from build123d import *

# Parameters (mm, degrees)
BOSS_EXTRUDE1_DEPTH = 12.7
SKETCH3_W           = 2.54
SKETCH3_H           = 5.08
CUT_EXTRUDE1_DEPTH  = 47.550334048
SKETCH4_W           = 55.88
SKETCH4_H           = 6.35
BOSS_EXTRUDE2_DEPTH = 26.67
SKETCH5_R           = 1.6
SKETCH5_W           = 31.75
SKETCH5_H           = 12.699510518
CUT_EXTRUDE3_DEPTH  = 89.325838235
CUT_EXTRUDE4_REACH  = 92.585
FILLET1_R           = 1.27
FILLET2_R           = 2.54


with BuildPart() as part:
    # Sketch2 → Boss-Extrude1 (new body)
    with BuildSketch(Plane.XY):
        with BuildLine():
            Line((-27.94, 0), (-10.7315, 0))
            ThreePointArc((-10.7315, 0), (0, -10.7315), (10.7315, 0))
            Line((10.7315, 0), (27.94, 0))
            Line((27.94, 0), (27.94, -35))
            Line((27.94, -35), (-27.94, -35))
            Line((-27.94, -35), (-27.94, 0))
        make_face()
    extrude(amount=BOSS_EXTRUDE1_DEPTH)

    # Sketch3 → Cut-Extrude1 (cut, through all)
    with BuildSketch(Plane(origin=(0, 0, 0), x_dir=(1, 0, 0), z_dir=(0, 1, 0))):
        with Locations((-21.423122, -6.35)):
            Rectangle(SKETCH3_W, SKETCH3_H)
        with Locations((21.423122, -6.35)):
            Rectangle(SKETCH3_W, SKETCH3_H)
    extrude(amount=-CUT_EXTRUDE1_DEPTH, mode=Mode.SUBTRACT)

    # Sketch4 → Boss-Extrude2 (add)
    with BuildSketch(Plane.XY.offset(12.7)):
        with Locations((0, -31.825)):
            Rectangle(SKETCH4_W, SKETCH4_H)
    extrude(amount=BOSS_EXTRUDE2_DEPTH)

    # Mirror1: part across plane


with BuildPart() as part_1:
    add(part.part)
    add(part.part.mirror(Plane(origin=(0, 0, 39.37), x_dir=(1, 0, 0), z_dir=(0, 0, -1))))

    # Sketch5 → Cut-Extrude3 (cut, through all)
    with BuildSketch(Plane(origin=(0, -28.65, 0), x_dir=(1, 0, 0), z_dir=(0, 1, 0))):
        with Locations(Location((-16.002, -28.87, 0), (0, 0, 270))):
            Circle(SKETCH5_R)
        with Locations(Location((-16.002, -49.87, 0), (0, 0, 270))):
            Circle(SKETCH5_R)
        with Locations((-6.985, -39.369755259)):
            Rectangle(SKETCH5_W, SKETCH5_H)
    extrude(amount=-CUT_EXTRUDE3_DEPTH, mode=Mode.SUBTRACT)

    # Cut-Extrude4: up to this face of the body (flat: up to its plane)
    cut_extrude4_end = Plane(part_1.part.faces().sort_by_distance((0, -18.819419433, 0))[0])
    # Sketch7 → Cut-Extrude4 (cut, up to the picked face)
    with BuildSketch(Plane.XY.offset(78.74), mode=Mode.PRIVATE) as cut_extrude4_sk1:
        with BuildLine():
            Line((0, -17.0815), (0, -35))
            Line((0, -35), (27.94, -35))
            Line((27.94, -35), (27.94, -6.35))
            Line((27.94, -6.35), (15.857337174, -6.35))
            ThreePointArc((15.857337174, -6.35), (9.573664848, -14.146468945), (0, -17.0815))
        make_face()
    cut_extrude4_tool1 = split(extrude(cut_extrude4_sk1.sketch, amount=-CUT_EXTRUDE4_REACH, mode=Mode.PRIVATE), bisect_by=cut_extrude4_end, keep=Keep.BOTH, mode=Mode.PRIVATE)
    add(cut_extrude4_tool1.solids().sort_by(Axis((15.36412, -22.474959, 78.74), (0, 0, -1)))[0], mode=Mode.SUBTRACT)

    # Fillet1
    fillet1_edges = [part_1.edges().sort_by_distance(p)[0] for p in [
        (-27.94, -35, 39.37),
        (22.693122, -6.35, 6.35),
        (22.693122, -6.35, 72.39),
        (27.94, -6.35, 72.39),
        (27.94, -6.35, 6.35),
        (-22.693122, -35, 6.35),
        (-22.693122, -35, 72.39),
    ]]
    fillet(fillet1_edges, radius=FILLET1_R)

    # Fillet2
    fillet2_edges = [part_1.edges().sort_by_distance(p)[0] for p in [
        (-22.86, -31.825, 45.719510518),
        (-22.86, -31.825, 33.02),
    ]]
    fillet(fillet2_edges, radius=FILLET2_R)


solid = part_1.part
Geometry: final body of the model. Coordinates: model frame, mm. A direction names the side the tool comes from. Round coordinates to 2 decimals unless told otherwise and drop trailing zeros. Order: outer loops, then holes, each group sorted by start corner. A loop starts at its lowest first (then second) coordinate and runs counter-clockwise, first axis right, second up. Notation, with made-up numbers: (41.5, 14.25) - (69.5, 14.25) arc R13 cw to (69.5, 38.25) - close; hole circle Ø10 at (-30.5, -30). An arc over 180 degrees is marked (long way). Write each question's results on one line, items separated by ' | '.
Item 1: Section C-C, the plane x = -3. Return the cut outline in (y, z), and give its area (3 significant figures).
Completed:
outline: (-35, 0) - (-10.3, 0) - (-10.3, 12.7) - (-28.65, 12.7) - (-28.65, 33.02) - (-35, 33.02) - close; (-35, 45.72) - (-28.65, 45.72) - (-28.65, 66.04) - (-10.3, 66.04) - (-10.3, 78.74) - (-35, 78.74) - close | area: 885 mm^2
Item 2: First-contact query: pin 1 Ø9 at (y, z) = (-25.5, 22) entering from +X; pin 2 Ø6 at (x, z) = (-17.5, 20.5) entering from +Y; pin 3 Ø8.5 at (x, z) = (19, 74.5) entering from -Y. Flat tips, straight axial feed; report the tip coordinate or a pass-through.
Completed:
pin 1: x = 0 | pin 2: y = -28.65 | pin 3: y = -8.61
Item 3: Section D-D, the plane z = 71.5. Return the cut outline in (x, y), and give its area (3 significant figures).
Completed:
outline: (-27.94, -33.73) arc R1.27 ccw to (-26.67, -35) - (-23.96, -35) arc R1.27 ccw to (-22.69, -33.73) - (-22.69, 0) - (-27.94, 0) - close; (-20.15, -35) - (0, -35) - (0, -17.08) arc R17.08 ccw to (15.86, -6.35) - (20.15, -6.35) - (20.15, 0) - (10.73, 0) arc R10.73 cw to (-10.73, 0) - (-20.15, 0) - close; (22.69, -5.08) arc R1.27 ccw to (23.96, -6.35) - (26.67, -6.35) arc R1.27 ccw to (27.94, -5.08) - (27.94, 0) - (22.69, 0) - close | area: 991 mm^2
Item 4: Mould query, pull axis X, two halves, no side actions, for faces 4 (the flat face through (-22, -17, 3.81)), 5 (the flat face through (-19, 0, 6)), 6 (the flat face through (-27.94, -32, 49)), 7 (the cylindrical face through (-22.136, -31.869, 33.784)). Classes: pulls with the +X half, pulls with the -X half, needs draft (parallel to the pull), parting line crosses it, or undercut.
Completed:
face 4: undercut | face 5: needs draft | face 6: pulls with the -X half | face 7: pulls with the +X half
Item 5: Section A-A, the plane y = -24. Return the cut outline in (x, z), and give its area (3 significant figures).
Completed:
outline: (-27.94, 0) - (0, 0) - (0, 12.7) - (-27.94, 12.7) - close; (-27.94, 66.04) - (0, 66.04) - (0, 78.74) - (-27.94, 78.74) - close; hole (-22.69, 3.81) - (-20.15, 3.81) - (-20.15, 8.89) - (-22.69, 8.89) - close; hole (-22.69, 69.85) - (-20.15, 69.85) - (-20.15, 74.93) - (-22.69, 74.93) - close | area: 684 mm^2
Item 6: Section B-B, the plane z = 28.87. Return the cut outline in (x, y), and give its area (3 significant figures).
Completed:
outline: (-27.94, -33.73) arc R1.27 ccw to (-26.67, -35) - (-17.6, -35) - (-17.6, -28.65) - (-27.94, -28.65) - close; (-14.4, -35) - (0, -35) - (0, -28.65) - (-14.4, -28.65) - close | area: 157 mm^2
Item 7: Material intervals for line 1 along Z through (x, y) = (-2, -32.5); line 2 along Z through (x, y) = (-9.5, -18); line 3 along X through (y, z) = (-25.5, 70), sorted ascending. Write a range as [from, to].
Completed:
line 1: [0, 33.02], [45.72, 78.74] | line 2: [0, 12.7], [66.04, 78.74] | line 3: [-27.94, -22.69], [-20.15, 0]
Item 8: Reachability of faces 1 (the cylindrical face through (-22.096, -31.869, 44.995)), 2 (the flat face through (0, -30, 13)), 3 (the flat face through (-6, -14, 12.7)) from +Z, -Z, +X, -X, +Y, -Y: full face, straight path, thin tool, end or side. Return the list, or none.
Completed:
face 1: +X, +Y, -Y | face 2: +Z, -Z, +X, -Y | face 3: +X, -X, +Y
